from build123d import *

# Parameters (mm, degrees)
SKETCH1_R           = 2.1
BOSS_EXTRUDE1_DEPTH = 1
FILLET1_R           = 1
BOSS_EXTRUDE2_DEPTH = 2.84
BOSS_EXTRUDE3_REACH = 76.197
SKETCH9_W           = 18
SKETCH9_H           = 10
SKETCH10_W          = 6.16
SKETCH10_H          = 10
SKETCH10_H_2        = 10.013009375
CUT_EXTRUDE1_DEPTH  = 6.1
BOSS_EXTRUDE4_START = -9
BOSS_EXTRUDE4_DEPTH = 18
CUT_EXTRUDE3_DEPTH  = 75.197102369
FILLET3_R           = 3
FILLET4_R           = 3
FILLET5_R           = 3
FILLET6_R           = 1
FILLET7_R           = 1


# Read off the part's stored shape, not the designer's step: Boss-Extrude4
with BuildPart() as part:
    # Sketch1 → Boss-Extrude1 (new body)
    with BuildSketch(Plane.XY):
        with BuildLine():
            Line((-2.839339828, 3.9), (-5.470710678, 6.53137085))
            ThreePointArc((-5.470710678, 6.53137085), (-5.492387953, 6.563813185), (-5.5, 6.602081528))
            Line((-5.5, 6.602081528), (-5.5, 8.1))
            ThreePointArc((-5.5, 8.1), (-5.470710678, 8.170710678), (-5.4, 8.2))
            Line((-5.4, 8.2), (-3.334418044, 8.2))
            ThreePointArc((-3.334418044, 8.2), (-3.244178397, 8.256909326), (-3.2566483, 8.362863876))
            Line((-3.2566483, 8.362863876), (-4.58, 10))
            Line((-4.58, 10), (-10, 10))
            Line((-10, 10), (-10, 4.58))
            Line((-10, 4.58), (-8.362863876, 3.2566483))
            ThreePointArc((-8.362863876, 3.2566483), (-8.256909326, 3.244178397), (-8.2, 3.334418044))
            Line((-8.2, 3.334418044), (-8.2, 5.4))
            ThreePointArc((-8.2, 5.4), (-8.170710678, 5.470710678), (-8.1, 5.5))
            Line((-8.1, 5.5), (-6.602081528, 5.5))
            ThreePointArc((-6.602081528, 5.5), (-6.563813185, 5.492387953), (-6.53137085, 5.470710678))
            Line((-6.53137085, 5.470710678), (-3.9, 2.839339828))
            Line((-3.9, 2.839339828), (-3.9, -2.839339828))
            Line((-3.9, -2.839339828), (-6.53137085, -5.470710678))
            ThreePointArc((-6.53137085, -5.470710678), (-6.563813185, -5.492387953), (-6.602081528, -5.5))
            Line((-6.602081528, -5.5), (-8.1, -5.5))
            ThreePointArc((-8.1, -5.5), (-8.170710678, -5.470710678), (-8.2, -5.4))
            Line((-8.2, -5.4), (-8.2, -3.334418044))
            ThreePointArc((-8.2, -3.334418044), (-8.256909326, -3.244178397), (-8.362863876, -3.2566483))
            Line((-8.362863876, -3.2566483), (-10, -4.58))
            Line((-10, -4.58), (-10, -10))
            Line((-10, -10), (-4.58, -10))
            Line((-4.58, -10), (-3.2566483, -8.362863876))
            ThreePointArc((-3.2566483, -8.362863876), (-3.244178397, -8.256909326), (-3.334418044, -8.2))
            Line((-3.334418044, -8.2), (-5.4, -8.2))
            ThreePointArc((-5.4, -8.2), (-5.470710678, -8.170710678), (-5.5, -8.1))
            Line((-5.5, -8.1), (-5.5, -6.602081528))
            ThreePointArc((-5.5, -6.602081528), (-5.492387953, -6.563813185), (-5.470710678, -6.53137085))
            Line((-5.470710678, -6.53137085), (-2.839339828, -3.9))
            Line((-2.839339828, -3.9), (2.839339828, -3.9))
            Line((2.839339828, -3.9), (5.470710678, -6.53137085))
            ThreePointArc((5.470710678, -6.53137085), (5.492387953, -6.563813185), (5.5, -6.602081528))
            Line((5.5, -6.602081528), (5.5, -8.1))
            ThreePointArc((5.5, -8.1), (5.470710678, -8.170710678), (5.4, -8.2))
            Line((5.4, -8.2), (3.334418044, -8.2))
            ThreePointArc((3.334418044, -8.2), (3.244178397, -8.256909326), (3.2566483, -8.362863876))
            Line((3.2566483, -8.362863876), (4.58, -10))
            Line((4.58, -10), (10, -10))
            Line((10, -10), (10, -4.58))
            Line((10, -4.58), (8.362863876, -3.2566483))
            ThreePointArc((8.362863876, -3.2566483), (8.256909326, -3.244178397), (8.2, -3.334418044))
            Line((8.2, -3.334418044), (8.2, -5.4))
            ThreePointArc((8.2, -5.4), (8.170710678, -5.470710678), (8.1, -5.5))
            Line((8.1, -5.5), (6.602081528, -5.5))
            ThreePointArc((6.602081528, -5.5), (6.563813185, -5.492387953), (6.53137085, -5.470710678))
            Line((6.53137085, -5.470710678), (3.9, -2.839339828))
            Line((3.9, -2.839339828), (3.9, 2.839339828))
            Line((3.9, 2.839339828), (6.53137085, 5.470710678))
            ThreePointArc((6.53137085, 5.470710678), (6.563813185, 5.492387953), (6.602081528, 5.5))
            Line((6.602081528, 5.5), (8.1, 5.5))
            ThreePointArc((8.1, 5.5), (8.170710678, 5.470710678), (8.2, 5.4))
            Line((8.2, 5.4), (8.2, 3.334418044))
            ThreePointArc((8.2, 3.334418044), (8.256909326, 3.244178397), (8.362863876, 3.2566483))
            Line((8.362863876, 3.2566483), (10, 4.58))
            Line((10, 4.58), (10, 10))
            Line((10, 10), (4.58, 10))
            Line((4.58, 10), (3.2566483, 8.362863876))
            ThreePointArc((3.2566483, 8.362863876), (3.244178397, 8.256909326), (3.334418044, 8.2))
            Line((3.334418044, 8.2), (5.4, 8.2))
            ThreePointArc((5.4, 8.2), (5.470710678, 8.170710678), (5.5, 8.1))
            Line((5.5, 8.1), (5.5, 6.602081528))
            ThreePointArc((5.5, 6.602081528), (5.492387953, 6.563813185), (5.470710678, 6.53137085))
            Line((5.470710678, 6.53137085), (2.839339828, 3.9))
            Line((2.839339828, 3.9), (-2.839339828, 3.9))
        make_face()
        Circle(SKETCH1_R, mode=Mode.SUBTRACT)
    extrude(amount=BOSS_EXTRUDE1_DEPTH)

    # Fillet1
    fillet1_edges = [part.edges().sort_by_distance(p)[0] for p in [
        (10, -10, 0.5),
        (-10, -10, 0.5),
        (-10, 10, 0.5),
        (10, 10, 0.5),
    ]]
    fillet(fillet1_edges, radius=FILLET1_R)


with BuildPart() as body_2:
    # 3DSketch1 → Boss-Extrude2 (new, symmetric)
    with BuildSketch(Plane(origin=(0, 3.9, 1), x_dir=(0, 0.7071067811865477, -0.7071067811865475), z_dir=(-1, 0, 0))):
        Polygon((0, 0), (70.710678119, 0), (35.355339059, 35.355339059), align=None)
    extrude(amount=BOSS_EXTRUDE2_DEPTH, both=True)

    # Boss-Extrude3: up to this plane
    boss_extrude3_end = Plane(origin=(2.84, 3.9, 1), z_dir=(0, 0.7071067811865475, 0.7071067811865476))
    # Sketch9 → Boss-Extrude3 (add, up to the surface)
    with BuildSketch(Plane(origin=(0, 0, -49), x_dir=(-1, 0, 0), z_dir=(0, 0, -1)), mode=Mode.PRIVATE) as boss_extrude3_sk1:
        with Locations((0, 15.013009375)):
            Rectangle(SKETCH9_W, SKETCH9_H)
    boss_extrude3_tool1 = split(extrude(boss_extrude3_sk1.sketch, amount=-BOSS_EXTRUDE3_REACH, mode=Mode.PRIVATE), bisect_by=boss_extrude3_end, keep=Keep.BOTH, mode=Mode.PRIVATE)
    add(boss_extrude3_tool1.solids().sort_by_distance((0, 15.013009, -49))[0])

    # Sketch10 → Cut-Extrude1 (cut)
    with BuildSketch(Plane(origin=(0, 0, -49), x_dir=(-1, 0, 0), z_dir=(0, 0, -1))):
        with Locations((-5.92, 15.013009375)):
            Rectangle(SKETCH10_W, SKETCH10_H)
        with Locations((5.92, 15.006504688)):
            Rectangle(SKETCH10_W, SKETCH10_H_2)
    extrude(amount=-CUT_EXTRUDE1_DEPTH, mode=Mode.SUBTRACT)

    # Boss-Extrude4 outline → Boss-Extrude4 (add)
    with BuildSketch(Plane.YZ.offset(BOSS_EXTRUDE4_START)):
        Polygon((20.013009375, -42.9), (47.8, -42.9), (37.8, -32.9), (20.013009375, -32.9), align=None)
    extrude(amount=BOSS_EXTRUDE4_DEPTH)


with BuildPart() as cut_extrude3_tool:
    # Sketch13 → Cut-Extrude3 (new, through all)
    with BuildSketch(Plane.XY.offset(1)):
        Polygon((-2.839339828, 3.9), (2.839339828, 3.9), (2.84, 10.013009375), (10.658445574, 10.013009375), (10.658445574, -10.0708852), (-2.84, -10.0708852), (-10.475035235, -10.0708852), (-10.475035235, 10.013009375), (-2.84, 10.013009375), align=None)
    extrude(amount=-CUT_EXTRUDE3_DEPTH)


with BuildPart() as part_1:
    add(part.part)

    # Cut-Extrude3: cut by cut_extrude3_tool
    add(cut_extrude3_tool.part, mode=Mode.SUBTRACT)


with BuildPart() as body_2_1:
    add(body_2.part)

    # Cut-Extrude3: cut by cut_extrude3_tool
    add(cut_extrude3_tool.part, mode=Mode.SUBTRACT)

    # Fillet3
    fillet3_edges = [body_2_1.edges().sort_by_distance(p)[0] for p in [
        (9, 20.013009375, -24.006504687),
    ]]
    fillet(fillet3_edges, radius=FILLET3_R)

    # Fillet4
    fillet4_edges = [body_2_1.edges().sort_by_distance(p)[0] for p in [
        (-9, 20.013009375, -24.006504687),
    ]]
    fillet(fillet4_edges, radius=FILLET4_R)

    # Fillet5
    fillet5_edges = [body_2_1.edges().sort_by_distance(p)[0] for p in [
        (9, 27.406504687, -32.9),
        (-9, 27.406504687, -32.9),
    ]]
    fillet(fillet5_edges, radius=FILLET5_R)

    # Fillet6
    fillet6_edges = [body_2_1.edges().sort_by_distance(p)[0] for p in [
        (0, 53.9, -49),
        (0, 3.9, 1),
    ]]
    fillet(fillet6_edges, radius=FILLET6_R)

    # Fillet7
    fillet7_edges = [body_2_1.edges().sort_by_distance(p)[0] for p in [
        (0, 3.9, -49),
    ]]
    fillet(fillet7_edges, radius=FILLET7_R)


solid = body_2_1.part
CAD build for the part. Positions are in the model's coordinates, mm. A direction names the side the tool comes from. Give positions to 0.01 mm unless a question says otherwise; leave off trailing zeros. Loops run counter-clockwise (first coordinate to the right, second up) from the corner with the lowest first, then second, coordinate; pieces in that order, holes last. Notation, with made-up numbers: M 8,20 L 61,20 A29 ccw 61,53 Z; hole C 21.5,31.25 d8. An arc over 180 degrees is marked long. Write each question's results on one line, items separated by ' | '.
Q1. Which spindle directions (+Z, -Z, +X, -X, +Y, -Y) get a long thin tool onto all of the face, cutting with end or side? Do faces 1 (the face through (4, 20.013, -24)), 2 (the face through (-4, 20.013, -24)), 3 (the face through (6, 29, -42.9)), 4 (the face through (6, 10.013, -24)). Say none if no direction does.
Geometry check:
face 1: +Z, +X, +Y | face 2: +Z, -X, +Y | face 3: -Z, +X, +Y, -Y | face 4: +Z, -Z, +X, -Y
Q2. Band-saw the part on D-D on z = -38. Write the cut outline in (x, y).
Geometry check:
outline: M -9,10.01 L -2.84,10.01 L -2.84,3.9 L 2.84,3.9 L 2.84,10.01 L 9,10.01 L 9,42.9 L -9,42.9 Z
Q3. Flat gauge pins, fed straight in: P1, Ø5, axis at x = -6.5, y = 24, coming from the -Z side; P2, Ø14, axis at y = 31, z = -28.5, coming from the -X side; P3, Ø7, axis at x = -6.5, z = -30, coming from the -Y side; P4, Ø5.5, axis at y = 31.5, z = -20, coming from the +X side. Where does each tip first touch, or does it go through?
Geometry check:
P1: stops at z = -42.9 | P2: stops at x = -8.97 | P3: stops at y = 10.01 | P4: passes through
Q4. Band-saw the part on B-B on z = -6. Write the cut outline in (x, y).
Geometry check:
outline: M -9,10.01 L -2.84,10.01 L -2.84,3.9 L 2.84,3.9 L 2.84,10.01 L 9,10.01 L 9,10.9 L -9,10.9 Z
Q5. Probe probe 1 along X at (y, z) = (45.5, -46); probe 2 along Z at (x, y) = (3, 34); probe 3 along Y at (x, z) = (4, -18). List the from-to ranges inside material, lowest first.
Geometry check:
probe 1: x = -2.84 to 2.84 | probe 2: z = -42.9 to -32.9 | probe 3: y = 10.01 to 20.01
Q6. Band-saw the part on C-C on x = 4.25. Write the cut outline in (y, z).
Geometry check:
outline: M 10.01,-42.9 L 47.8,-42.9 L 37.8,-32.9 L 20.01,-32.9 L 20.01,-15.11 L 10.01,-5.11 Z
Q7. Band-saw the part on A-A on y = 30.5. Write the cut outline in (x, z), and give its area (3 significant figures).
Geometry check:
outline: M -9,-42.9 L -2.84,-42.9 L -2.84,-49 L 2.84,-49 L 2.84,-42.9 L 9,-42.9 L 9,-35.9 A3 ccw 6,-32.9 L 2.84,-32.9 L 2.84,-25.6 L -2.84,-25.6 L -2.84,-32.9 L -6,-32.9 A3 ccw -9,-35.9 Z | area: 252 mm²
